Read the model definition and answer for the solid it produces. Units are mm, in the model's axes. Face numbers are marked on the shaded views. Give positions to 0.01 mm unless a question says otherwise; leave off trailing zeros. Order: outer loops, then holes, each group sorted by start corner. A loop starts at its lowest first (then second) coordinate and runs counter-clockwise, first axis right, second up. Notation, with made-up numbers: (2, 15) - (32, 15) arc R20 ccw to (32, 52) - close; hole circle Ø2 at (-8.75, 89). An arc over 180 degrees is marked (long way). Return JSON: item names as keys, results as strings.
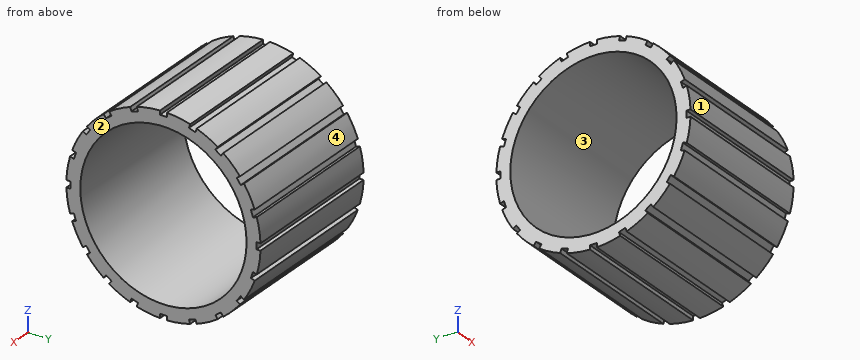
```python
from build123d import *

# Parameters (mm, degrees)
F0_W     = 110
F0_H     = 10.264
F3_DEPTH = 110


with BuildPart() as f1:
    # F0 (on Top) → F1 (revolve)
    with BuildSketch(Plane.XY):
        with Locations((0, 66.242)):
            Rectangle(F0_W, F0_H)
    revolve(axis=Axis((32.912049, 0, 0), (1, 0, 0)))

    # F2 (on face) → F3 (cut, through all)
    with BuildSketch(Plane.YZ.offset(55)):
        with BuildLine():
            ThreePointArc((2.5, 71.330203), (1.250192, 71.36305), (0, 71.374))
            ThreePointArc((0, 71.374), (-1.250192, 71.36305), (-2.5, 71.330203))
            Line((-2.5, 71.330203), (-2.5, 68.374))
            Line((-2.5, 68.374), (2.5, 68.374))
            Line((2.5, 68.374), (2.5, 71.330203))
        make_face()
        with BuildLine():
            ThreePointArc((22.055779, 67.880708), (20.863392, 68.256624), (19.664604, 68.611597))
            Line((19.664604, 68.611597), (18.751087, 65.800081))
            Line((18.751087, 65.800081), (23.506369, 64.254996))
            Line((23.506369, 64.254996), (24.419886, 67.066512))
            ThreePointArc((24.419886, 67.066512), (23.241398, 67.483963), (22.055779, 67.880708))
        make_face()
        with BuildLine():
            ThreePointArc((41.952585, 57.742779), (40.934722, 58.468764), (39.904299, 59.17681))
            Line((39.904299, 59.17681), (38.166686, 56.785191))
            Line((38.166686, 56.785191), (42.211771, 53.846265))
            Line((42.211771, 53.846265), (43.949384, 56.237883))
            ThreePointArc((43.949384, 56.237883), (42.957575, 56.999076), (41.952585, 57.742779))
        make_face()
        with BuildLine():
            ThreePointArc((57.742779, 41.952585), (56.999076, 42.957575), (56.237883, 43.949384))
            Line((56.237883, 43.949384), (53.846265, 42.211771))
            Line((53.846265, 42.211771), (56.785191, 38.166686))
            Line((56.785191, 38.166686), (59.17681, 39.904299))
            ThreePointArc((59.17681, 39.904299), (58.468765, 40.934722), (57.742779, 41.952585))
        make_face()
        with BuildLine():
            ThreePointArc((67.880708, 22.055779), (67.483963, 23.241398), (67.066512, 24.419886))
            Line((67.066512, 24.419886), (64.254996, 23.506369))
            Line((64.254996, 23.506369), (65.800081, 18.751087))
            Line((65.800081, 18.751087), (68.611597, 19.664604))
            ThreePointArc((68.611597, 19.664604), (68.256624, 20.863392), (67.880708, 22.055779))
        make_face()
        with BuildLine():
            ThreePointArc((71.374, 0), (71.36305, 1.250192), (71.330203, 2.5))
            Line((71.330203, 2.5), (68.374, 2.5))
            Line((68.374, 2.5), (68.374, -2.5))
            Line((68.374, -2.5), (71.330203, -2.5))
            ThreePointArc((71.330203, -2.5), (71.36305, -1.250192), (71.374, 0))
        make_face()
        with BuildLine():
            ThreePointArc((67.880708, -22.055779), (68.256624, -20.863392), (68.611597, -19.664604))
            Line((68.611597, -19.664604), (65.800081, -18.751087))
            Line((65.800081, -18.751087), (64.254996, -23.506369))
            Line((64.254996, -23.506369), (67.066512, -24.419886))
            ThreePointArc((67.066512, -24.419886), (67.483963, -23.241398), (67.880708, -22.055779))
        make_face()
        with BuildLine():
            ThreePointArc((57.742779, -41.952584), (58.468765, -40.934722), (59.17681, -39.904299))
            Line((59.17681, -39.904299), (56.785191, -38.166686))
            Line((56.785191, -38.166686), (53.846265, -42.211771))
            Line((53.846265, -42.211771), (56.237883, -43.949384))
            ThreePointArc((56.237883, -43.949384), (56.999076, -42.957575), (57.742779, -41.952584))
        make_face()
        with BuildLine():
            ThreePointArc((41.952585, -57.742779), (42.957575, -56.999076), (43.949384, -56.237883))
            Line((43.949384, -56.237883), (42.211771, -53.846265))
            Line((42.211771, -53.846265), (38.166686, -56.785191))
            Line((38.166686, -56.785191), (39.904299, -59.17681))
            ThreePointArc((39.904299, -59.17681), (40.934722, -58.468764), (41.952585, -57.742779))
        make_face()
        with BuildLine():
            ThreePointArc((22.055779, -67.880708), (23.241398, -67.483963), (24.419886, -67.066512))
            Line((24.419886, -67.066512), (23.506369, -64.254996))
            Line((23.506369, -64.254996), (18.751087, -65.800081))
            Line((18.751087, -65.800081), (19.664604, -68.611597))
            ThreePointArc((19.664604, -68.611597), (20.863392, -68.256624), (22.055779, -67.880708))
        make_face()
        with BuildLine():
            Line((-2.5, -68.374), (-2.5, -71.330203))
            ThreePointArc((-2.5, -71.330203), (-1.250192, -71.36305), (0, -71.374))
            ThreePointArc((0, -71.374), (1.250192, -71.36305), (2.5, -71.330203))
            Line((2.5, -71.330203), (2.5, -68.374))
            Line((2.5, -68.374), (-2.5, -68.374))
        make_face()
        with BuildLine():
            Line((-23.506369, -64.254996), (-24.419886, -67.066512))
            ThreePointArc((-24.419886, -67.066512), (-23.241398, -67.483963), (-22.055779, -67.880708))
            ThreePointArc((-22.055779, -67.880708), (-20.863392, -68.256624), (-19.664604, -68.611597))
            Line((-19.664604, -68.611597), (-18.751087, -65.800081))
            Line((-18.751087, -65.800081), (-23.506369, -64.254996))
        make_face()
        with BuildLine():
            Line((-42.211771, -53.846265), (-43.949384, -56.237883))
            ThreePointArc((-43.949384, -56.237883), (-42.957575, -56.999076), (-41.952585, -57.742779))
            ThreePointArc((-41.952585, -57.742779), (-40.934722, -58.468764), (-39.904299, -59.17681))
            Line((-39.904299, -59.17681), (-38.166686, -56.785191))
            Line((-38.166686, -56.785191), (-42.211771, -53.846265))
        make_face()
        with BuildLine():
            Line((-56.785191, -38.166686), (-59.17681, -39.904299))
            ThreePointArc((-59.17681, -39.904299), (-58.468764, -40.934722), (-57.742779, -41.952585))
            ThreePointArc((-57.742779, -41.952585), (-56.999076, -42.957575), (-56.237883, -43.949384))
            Line((-56.237883, -43.949384), (-53.846265, -42.211771))
            Line((-53.846265, -42.211771), (-56.785191, -38.166686))
        make_face()
        with BuildLine():
            Line((-65.800081, -18.751087), (-68.611597, -19.664604))
            ThreePointArc((-68.611597, -19.664604), (-68.256624, -20.863392), (-67.880708, -22.055779))
            ThreePointArc((-67.880708, -22.055779), (-67.483963, -23.241398), (-67.066512, -24.419886))
            Line((-67.066512, -24.419886), (-64.254996, -23.506369))
            Line((-64.254996, -23.506369), (-65.800081, -18.751087))
        make_face()
        with BuildLine():
            Line((-68.374, 2.5), (-71.330203, 2.5))
            ThreePointArc((-71.330203, 2.5), (-71.36305, 1.250192), (-71.374, 0))
            ThreePointArc((-71.374, 0), (-71.36305, -1.250192), (-71.330203, -2.5))
            Line((-71.330203, -2.5), (-68.374, -2.5))
            Line((-68.374, -2.5), (-68.374, 2.5))
        make_face()
        with BuildLine():
            Line((-64.254996, 23.506369), (-67.066512, 24.419886))
            ThreePointArc((-67.066512, 24.419886), (-67.483963, 23.241399), (-67.880708, 22.05578))
            ThreePointArc((-67.880708, 22.05578), (-68.256624, 20.863392), (-68.611597, 19.664604))
            Line((-68.611597, 19.664604), (-65.800081, 18.751087))
            Line((-65.800081, 18.751087), (-64.254996, 23.506369))
        make_face()
        with BuildLine():
            Line((-53.846265, 42.211771), (-56.237883, 43.949384))
            ThreePointArc((-56.237883, 43.949384), (-56.999076, 42.957575), (-57.742779, 41.952585))
            ThreePointArc((-57.742779, 41.952585), (-58.468764, 40.934722), (-59.17681, 39.904299))
            Line((-59.17681, 39.904299), (-56.785191, 38.166686))
            Line((-56.785191, 38.166686), (-53.846265, 42.211771))
        make_face()
        with BuildLine():
            Line((-38.166686, 56.785191), (-39.904299, 59.17681))
            ThreePointArc((-39.904299, 59.17681), (-40.934722, 58.468764), (-41.952585, 57.742779))
            ThreePointArc((-41.952585, 57.742779), (-42.957575, 56.999076), (-43.949384, 56.237883))
            Line((-43.949384, 56.237883), (-42.211771, 53.846265))
            Line((-42.211771, 53.846265), (-38.166686, 56.785191))
        make_face()
        with BuildLine():
            Line((-18.751087, 65.800081), (-19.664604, 68.611597))
            ThreePointArc((-19.664604, 68.611597), (-20.863392, 68.256624), (-22.055779, 67.880708))
            ThreePointArc((-22.055779, 67.880708), (-23.241398, 67.483963), (-24.419886, 67.066512))
            Line((-24.419886, 67.066512), (-23.506369, 64.254996))
            Line((-23.506369, 64.254996), (-18.751087, 65.800081))
        make_face()
    extrude(amount=-F3_DEPTH, mode=Mode.SUBTRACT)


solid = f1.part
```
Q1. Given pin 1 (1 mm diameter, centred on x = -43.5, z = 31.5, fed in from +Y); pin 2 (12 mm diameter, centred on x = -9, z = -31, fed in from -Y); pin 3 (2.5 mm diameter, centred on x = 15, z = 1, fed in from -Y); pin 4 (5.5 mm diameter, centred on x = 1.5, z = 1, fed in from +Y), each flat-ended and moving along its own axis, determine where each tip first touches the part or whether it passes through.
Values:
{"pin 1": "stops at y = 64.29", "pin 2": "stops at y = -66.85", "pin 3": "stops at y = -68.37", "pin 4": "stops at y = 71.33"}
Q2. A cutting plane is placed at A-A (z = 0). Write down the section's boundary in (x, y).
Values:
{"outline": "(-55, -68.37) - (55, -68.37) - (55, -61.11) - (-55, -61.11) - close; (-55, 61.11) - (55, 61.11) - (55, 68.37) - (-55, 68.37) - close"}
Q3. Determine the mould class of the marked faces 1, 2, 3 and 4 for opening direction Y: released by +Y, released by -Y, zero draft, split by the parting line, or undercut.
Values:
{"face 1": "released by -Y", "face 2": "zero draft", "face 3": "undercut", "face 4": "released by +Y"}
Q4. Consider L1, parallel to Z at x = -31.5, y = 0; L2, parallel to Z at x = -22, y = -55.5; L3, parallel to Z at x = 34, y = -41. Determine where each line is inside the solid, lowest interval first.
Values:
{"L1": "z = -68.37 to -61.11, 61.11 to 68.37", "L2": "z = -44.88 to -43.41, -39.94 to -25.58, 25.58 to 39.94, 43.41 to 44.88", "L3": "z = -54.73 to -45.31, 45.31 to 54.73"}
